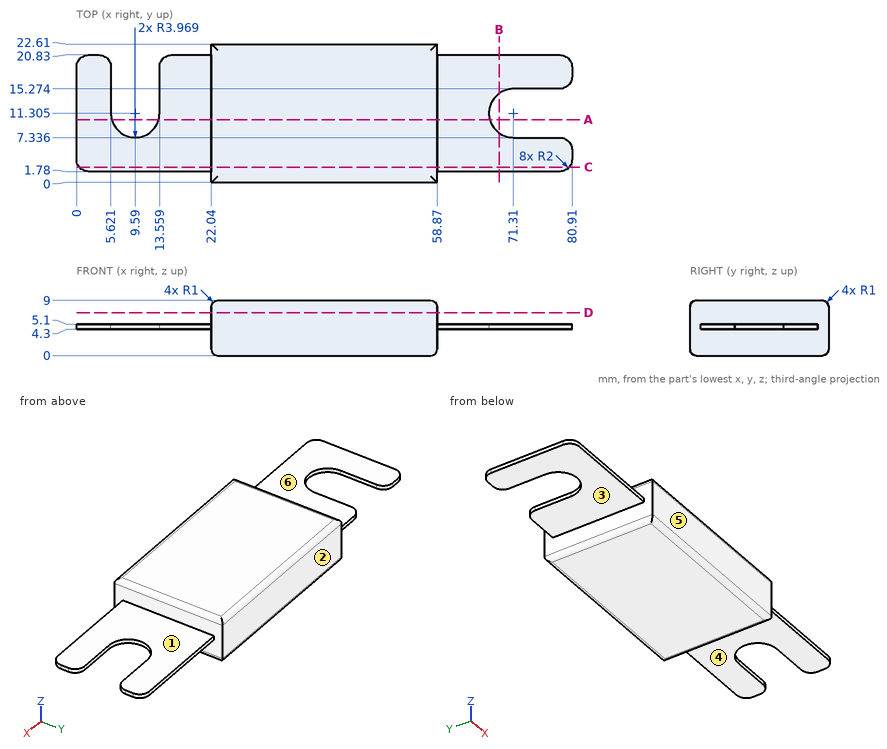
Design review of the part shown in the three views and the two pictorial views. Dimensions are in mm from the part's minimum x, y and z. A direction names the side the tool comes from. Give positions to 0.01 mm unless a question says otherwise; leave off trailing zeros. Write each loop counter-clockwise with the first axis right and the second up, starting at its lowest first coordinate (ties: lowest second). Pieces come first, ordered by that corner, then holes. Notation, with made-up numbers: M -16.75,42.25 L 0.25,42.25 A4 cw 0.25,47.25 Z; hole C 83.25,-24.75 d3. An arc over 180 degrees is marked long. Answer in a Markdown table with one row per item.
Item 1: Tool access review of the marked faces 4, 5 and 6: name each direction out of +Z, -Z, +X, -X, +Y, -Y from which nothing blocks a thin tool from reaching the whole face with its end or side.
Check sheet entries:
| item | result |
|---|---|
| face 4 | -Z, +X, +Y, -Y |
| face 5 | +Z, -Z, +X, -X, -Y |
| face 6 | +Z, -X, +Y, -Y |
Item 2: For P1, Ø0.9, axis at x = 65.5, z = 5, coming from the +Y side; P2, Ø5.5, axis at x = 66.5, y = 14.5, coming from the +Z side; P3, Ø5.5, axis at x = 8.5, y = 10, coming from the -Z side; P4, Ø5, axis at x = 66.5, z = 1.5, coming from the -Y side (1 decimal), all flat-tipped, find the tip position at first contact; note any pin that passes through.
Check sheet entries:
| item | result |
|---|---|
| P1 | y = 20.83 |
| P2 | z = 5.1 |
| P3 | z = 4.3 |
| P4 | through |
Item 3: Add section C-C on y = 2.5. Give the boundary of the cut face in (x, z), plus the area to 3 significant figures.
Check sheet entries:
| item | result |
|---|---|
| outline | M 0.46,4.3 L 22.04,4.3 L 22.04,1 A1 ccw 23.04,0 L 57.87,0 A1 ccw 58.87,1 L 58.87,4.3 L 80.45,4.3 L 80.45,5.1 L 58.87,5.1 L 58.87,8 A1 ccw 57.87,9 L 23.04,9 A1 ccw 22.04,8 L 22.04,5.1 L 0.46,5.1 Z |
| area | 365 mm2 |
Item 4: Add section D-D on z = 7. Give the boundary of the cut face in (x, y), plus the area to 3 significant figures.
Check sheet entries:
| item | result |
|---|---|
| outline | M 22.04,0 L 58.87,0 L 58.87,22.61 L 22.04,22.61 Z |
| area | 833 mm2 |
Item 5: Add section B-B on x = 69. Give the boundary of the cut face in (y, z), plus the area to 3 significant figures.
Check sheet entries:
| item | result |
|---|---|
| outline | M 1.78,4.3 L 8.08,4.3 L 8.08,5.1 L 1.78,5.1 Z; M 14.53,4.3 L 20.83,4.3 L 20.83,5.1 L 14.53,5.1 Z |
| area | 10.1 mm2 |
Item 6: For line 1 along Z through (x, y) = (17.5, 8.75); line 2 along X through (y, z) = (7.5, 7.5); line 3 along Y through (x, z) = (18, 5), list the stretches that pass through material, from the lowest coordinate up.
Check sheet entries:
| item | result |
|---|---|
| line 1 | 4.3 to 5.1 |
| line 2 | 22.04 to 58.87 |
| line 3 | 1.78 to 20.83 |
Item 7: Add section A-A on y = 10.25. Give the boundary of the cut face in (x, z), plus the area to 3 significant figures.
Check sheet entries:
| item | result |
|---|---|
| outline | M 0,4.3 L 5.76,4.3 L 5.76,5.1 L 0,5.1 Z; M 13.42,4.3 L 22.04,4.3 L 22.04,1 A1 ccw 23.04,0 L 57.87,0 A1 ccw 58.87,1 L 58.87,4.3 L 67.48,4.3 L 67.48,5.1 L 58.87,5.1 L 58.87,8 A1 ccw 57.87,9 L 23.04,9 A1 ccw 22.04,8 L 22.04,5.1 L 13.42,5.1 Z |
| area | 349 mm2 |
Item 8: Draft analysis for pull direction Z (two halves, no side actions). For the marked faces 1, 2 and 3, state which applies: +Z half, -Z half, draft (parallel to the pull), parting line (faces both ways), or undercut.
Check sheet entries:
| item | result |
|---|---|
| face 1 | +Z half |
| face 2 | draft |
| face 3 | -Z half |
